Source: CAD feature listing. Evaluate the final solid. Frame: model axes, mm. A direction names the side the tool comes from. Round coordinates to 2 decimals unless told otherwise and drop trailing zeros. Write each loop counter-clockwise with the first axis right and the second up, starting at its lowest first coordinate (ties: lowest second). Pieces come first, ordered by that corner, then holes. Notation, with made-up numbers: M 89,28.25 L 106,28.25 A23 cw 106,38.25 Z; hole C 5.5,-19 d7. An arc over 180 degrees is marked long. Use a Markdown table: item, result.
```python
from build123d import *

# Parameters (mm, degrees)
SKETCH_1_W               = 600
SKETCH_1_H               = 1200
EXTRUDE_1_DEPTH          = 2000
SKETCH_2_R               = 25
EXTRUDE_2_DEPTH          = 80
MIRROR_2_COPY_1_SKETCH_R = 25
MIRROR_2_COPY_1_DEPTH    = 80
SKETCH_3_W               = 525
SKETCH_3_H               = 1260
EXTRUDE_3_DEPTH          = 5


with BuildPart() as part:
    # 草图1 → 凸台-拉伸1 (new body)
    with BuildSketch(Plane(origin=(0, 0, 0), x_dir=(1, 0, 0), z_dir=(0, 1, 0))):
        Rectangle(SKETCH_1_W, SKETCH_1_H)
    extrude(amount=EXTRUDE_1_DEPTH)

    # 草图2 → 凸台-拉伸2 (add)
    with BuildSketch(Plane.XZ):
        with Locations((275, 575)):
            Circle(SKETCH_2_R)
    extrude_2 = extrude(amount=EXTRUDE_2_DEPTH)

    # 镜向1: 凸台-拉伸2 across plane
    add(extrude_2.mirror(Plane(origin=(0, 0, 0), x_dir=(0, 0, 1), z_dir=(1, 0, 0))))

    # 镜向2: 凸台-拉伸2 across plane
    add(extrude_2.mirror(Plane.XY))

    # 镜向2 copy 1 sketch → 镜向2 copy 1 (add)
    with BuildSketch(Plane(origin=(0, 0, 0), x_dir=(-1, 0, 0), z_dir=(0, -1, 0))):
        with Locations((275, 575)):
            Circle(MIRROR_2_COPY_1_SKETCH_R)
    extrude(amount=MIRROR_2_COPY_1_DEPTH)

    # 草图3 → 凸台-拉伸3 (add)
    with BuildSketch(Plane(origin=(300, 0, 0), x_dir=(0, 0, -1), z_dir=(1, 0, 0))):
        with Locations((-287.5, 1320)):
            Rectangle(SKETCH_3_W, SKETCH_3_H)
    extrude_3 = extrude(amount=EXTRUDE_3_DEPTH)

    # 镜向3: 凸台-拉伸3 across plane
    add(extrude_3.mirror(Plane.XY))


solid = part.part
```
Q1. Section A-A on z = 390. Return loops of the section in (x, y), plus the area to 3 significant figures.
Results are:
| item | result |
|---|---|
| outline | M -300,0 L 300,0 L 300,690 L 305,690 L 305,1950 L 300,1950 L 300,2000 L -300,2000 Z |
| area | 1,210,000 mm^2 |
Q2. Mould query, pull axis X, two halves, no side actions, for faces 1 (the flat face through (-4, 986, -600)), 2 (the flat face through (305, 1329, -291)), 3 (the cylindrical face through (-298.846, -39.44, -582.509)). Classes: +X half, -X half, draft (parallel to the pull), parting line (faces both ways), or undercut.
Results are:
| item | result |
|---|---|
| face 1 | draft |
| face 2 | +X half |
| face 3 | undercut |
Q3. Reachability of faces 4 (the cylindrical face through (298.846, -39.44, 582.509)), 5 (the flat face through (-275, -80, 575)) from +Z, -Z, +X, -X, +Y, -Y: full face, straight path, thin tool, end or side. Return the list, or none.
Results are:
| item | result |
|---|---|
| face 4 | -Y |
| face 5 | +Z, -Z, +X, -X, -Y |
Q4. Section B-B on x = 58.5. Return loops of the section in (y, z).
Results are:
| item | result |
|---|---|
| outline | M 0,-600 L 2000,-600 L 2000,600 L 0,600 Z |
Q5. Line query: L1, parallel to Y at x = 34, z = 163.5; L2, parallel to X at y = 545.5, z = -89. Output: solid intervals per line, ascending.
Results are:
| item | result |
|---|---|
| L1 | 0 to 2000 |
| L2 | -300 to 300 |
Q6. First-contact query: pin 1 Ø2.5 at (x, y) = (301.5, 1147) entering from -Z; pin 2 Ø1.5 at (x, z) = (302, -224.5) entering from +Y; pin 3 Ø1 at (y, z) = (511.5, -96) entering from +X. Flat tips, straight axial feed; report the tip coordinate or a pass-through.
Results are:
| item | result |
|---|---|
| pin 1 | z = -550 |
| pin 2 | y = 1950 |
| pin 3 | x = 300 |
